Design review of the part built by this model. Coordinates are the model's own, in mm. Coordinates: 2 decimals unless noted, no trailing zeros. Write each loop counter-clockwise with the first axis right and the second up, starting at its lowest first coordinate (ties: lowest second). Pieces come first, ordered by that corner, then holes.
Q1. Add section C-C, the plane z = 2.7. Give the boundary of the cut face in (x, y), plus the area to 3 significant figures.
Q2. The part is to be moulded in two halves that separate along X. For faces 1 (the face through (174, 115, 2)), 2 (the face through (79, 65, 0)), 3 (the face through (85.6, 168.3, 1)), 4 (the face through (-2, 115, 2)), say which applies: +X half, -X half, draft (parallel to the pull), parting line (faces both ways), or undercut.
Q3. To check wall thickness, follow probe 1 along X at (y, z) = (132, 0.85); probe 2 along X at (y, z) = (149.5, 2.15); probe 3 along Y at (x, z) = (48, 1.35). State the ranges of each line that lie inside material, in increasing order.
Q4. Add section D-D, the plane x = 86. Give the boundary of the cut face in (y, z), plus the area to 3 significant figures.
Q5. Add section B-B, the plane y = 91. Give the boundary of the cut face in (x, z), plus the area to 3 significant figures.
Q6. Add section A-A, the plane x = 133. Give the boundary of the cut face in (y, z).
from build123d import *

# Parameters (mm, degrees)
SKETCH025_W     = 176
SKETCH025_H     = 115
SKETCH025_W_2   = 166
SKETCH025_H_2   = 99
PAD009_DEPTH    = 2
SKETCH026_W     = 170
SKETCH026_H     = 103
POCKET012_DEPTH = 1
SKETCH027_W     = 176
SKETCH027_H     = 115
SKETCH027_W_2   = 172
SKETCH027_H_2   = 111
PAD010_DEPTH    = 3.5
SKETCH028_W     = 24
SKETCH028_H     = 15
POCKET013_DEPTH = 1.5


with BuildPart() as part:
    # Sketch025 → Pad009 (new body)
    with BuildSketch(Plane.XY):
        with Locations((86, 115.5)):
            Rectangle(SKETCH025_W, SKETCH025_H)
        with Locations((86, 118.5)):
            Rectangle(SKETCH025_W_2, SKETCH025_H_2, mode=Mode.SUBTRACT)
    extrude(amount=PAD009_DEPTH)

    # Sketch026 → Pocket012 (cut)
    with BuildSketch(Plane.XY.offset(2)):
        with Locations((86, 118.5)):
            Rectangle(SKETCH026_W, SKETCH026_H)
    extrude(amount=-POCKET012_DEPTH, mode=Mode.SUBTRACT)

    # Sketch027 → Pad010 (join)
    with BuildSketch(Plane.XY):
        with Locations((86, 115.5)):
            Rectangle(SKETCH027_W, SKETCH027_H)
        with Locations((86, 115.5)):
            Rectangle(SKETCH027_W_2, SKETCH027_H_2, mode=Mode.SUBTRACT)
    extrude(amount=PAD010_DEPTH)

    # Sketch028 → Pocket013 (cut)
    with BuildSketch(Plane.XY.offset(3.5)):
        with Locations((85, 53.5)):
            Rectangle(SKETCH028_W, SKETCH028_H)
    extrude(amount=-POCKET013_DEPTH, mode=Mode.SUBTRACT)


solid = part.part
Here are the results:
1. outline: (-2, 58) - (73, 58) - (73, 60) - (0, 60) - (0, 171) - (172, 171) - (172, 60) - (97, 60) - (97, 58) - (174, 58) - (174, 173) - (-2, 173) - close
1. area: 1,100 mm2
2. face 1: +X half
2. face 2: draft
2. face 3: undercut
2. face 4: -X half
3. probe 1: x = -2 to 3, 169 to 174
3. probe 2: x = -2 to 0, 172 to 174
3. probe 3: y = 58 to 67, 170 to 173
4. outline: (58, 0) - (69, 0) - (69, 1) - (67, 1) - (67, 2) - (58, 2) - close; (168, 0) - (173, 0) - (173, 3.5) - (171, 3.5) - (171, 2) - (170, 2) - (170, 1) - (168, 1) - close
4. area: 31.0 mm2
5. outline: (-2, 0) - (3, 0) - (3, 1) - (1, 1) - (1, 2) - (0, 2) - (0, 3.5) - (-2, 3.5) - close; (169, 0) - (174, 0) - (174, 3.5) - (172, 3.5) - (172, 2) - (171, 2) - (171, 1) - (169, 1) - close
5. area: 22.0 mm2
6. outline: (58, 0) - (69, 0) - (69, 1) - (67, 1) - (67, 2) - (60, 2) - (60, 3.5) - (58, 3.5) - close; (168, 0) - (173, 0) - (173, 3.5) - (171, 3.5) - (171, 2) - (170, 2) - (170, 1) - (168, 1) - close
